Geometry: final body of the model. Coordinates: model frame, mm. A direction names the side the tool comes from. Round coordinates to 2 decimals unless told otherwise and drop trailing zeros. Loops run counter-clockwise (first coordinate to the right, second up) from the corner with the lowest first, then second, coordinate; pieces in that order, holes last. Notation, with made-up numbers: M -29.5,13 L -13.5,13 A18 ccw -13.5,30 Z; hole C -3.75,26 d2. An arc over 180 degrees is marked long. Answer as a JSON object with one key per item and string values.
```python
from build123d import *

# Parameters (mm, degrees)
F1_DEPTH = 1.5
F3_DEPTH = 1
F4_R     = 1.3
F5_DEPTH = 25


with BuildPart() as f1:
    # F0 (on Top) → F1 (new body)
    with BuildSketch(Plane.XY):
        with BuildLine():
            Line((-2, 0), (0, 0))
            Line((0, 0), (2, 0))
            ThreePointArc((2, 0), (2.8640349955, 2.0859650045), (4.95, 2.95))
            Line((4.95, 2.95), (-4.95, 2.95))
            ThreePointArc((-4.95, 2.95), (-2.8640349955, 2.0859650045), (-2, 0))
        make_face()
        with BuildLine():
            Line((2, 0), (0, 0))
            Line((0, 0), (-2, 0))
            ThreePointArc((-2, 0), (-2.8640349955, -2.0859650045), (-4.95, -2.95))
            Line((-4.95, -2.95), (4.95, -2.95))
            ThreePointArc((4.95, -2.95), (2.8640349955, -2.0859650045), (2, 0))
        make_face()
        with BuildLine():
            ThreePointArc((4.95, 2.95), (2.8640349955, 2.0859650045), (2, 0))
            Line((2, 0), (4.95, 0))
            Line((4.95, 0), (4.95, 2.95))
        make_face()
        with BuildLine():
            Line((4.95, 0), (2, 0))
            ThreePointArc((2, 0), (2.8640349955, -2.0859650045), (4.95, -2.95))
            ThreePointArc((4.95, -2.95), (7.0359650045, -2.0859650045), (7.9, 0))
            ThreePointArc((7.9, 0), (7.0359650045, 2.0859650045), (4.95, 2.95))
            Line((4.95, 2.95), (4.95, 0))
        make_face()
        with BuildLine():
            ThreePointArc((-4.95, -2.95), (-2.8640349955, -2.0859650045), (-2, 0))
            ThreePointArc((-2, 0), (-2.8640349955, 2.0859650045), (-4.95, 2.95))
            ThreePointArc((-4.95, 2.95), (-7.9, 0), (-4.95, -2.95))
        make_face()
    extrude(amount=F1_DEPTH)

    # F2 (on face) → F3 (cut)
    with BuildSketch(Plane(origin=(0, 0, 0), x_dir=(1, 0, 0), z_dir=(0, 0, -1))):
        Polygon((1.3, -2.2516660498), (2.6, 0), (1.3, 2.2516660498), (-1.3, 2.2516660498), (-2.6, 0), (-1.3, -2.2516660498), align=None)
    extrude(amount=-F3_DEPTH, mode=Mode.SUBTRACT)

    # F4 (on face) → F5 (cut)
    with BuildSketch(Plane(origin=(0, 0, 1), x_dir=(1, 0, 0), z_dir=(0, 0, -1))):
        Circle(F4_R)
    extrude(amount=-F5_DEPTH, mode=Mode.SUBTRACT)


solid = f1.part
```
1) Cut plane A-A on z = 0.35. Return the cut outline in (x, y).
Geometry results:
{"outline": "M -4.95,-2.95 L 4.95,-2.95 A2.95 ccw 4.95,2.95 L -4.95,2.95 A2.95 ccw Z; hole M -2.6,0 L -1.3,-2.25 L 1.3,-2.25 L 2.6,0 L 1.3,2.25 L -1.3,2.25 Z"}
2) Line query: probe 1 along X at (y, z) = (0, 1.45); probe 2 along Y at (x, z) = (0, 1.35); probe 3 along Y at (x, z) = (1, 0.95). Output: solid intervals per line, ascending.
Geometry results:
{"probe 1": "-7.9 to -1.3, 1.3 to 7.9", "probe 2": "-2.95 to -1.3, 1.3 to 2.95", "probe 3": "-2.95 to -2.25, 2.25 to 2.95"}
3) Cut plane C-C on y = 0.3. Return the cut outline in (x, z).
Geometry results:
{"outline": "M -7.88,0 L -2.43,0 L -2.43,1 L -1.26,1 L -1.26,1.5 L -7.88,1.5 Z; M 1.26,1 L 2.43,1 L 2.43,0 L 7.88,0 L 7.88,1.5 L 1.26,1.5 Z"}
4) Pull-direction query (Y, two-part tool) for faces 1 (the face through (0, 2.95, 1)), 2 (the face through (0, -2.95, 1)), 3 (the face through (1.96, -1.11, 0.49)), 4 (the face through (7.9, -0.1, 0.7)); classes: +Y half, -Y half, draft (parallel to the pull), parting line (faces both ways), or undercut.
Geometry results:
{"face 1": "+Y half", "face 2": "-Y half", "face 3": "undercut", "face 4": "parting line"}
5) Set-up query: faces 5 (the face through (1.94, 1.14, 0.49)), 6 (the face through (2, -2, 0)). Return all of +Z, -Z, +X, -X, +Y, -Y with unobstructed straight access to the full face (end or side cutting, diameter ignored); none if empty.
Geometry results:
{"face 5": "-Z", "face 6": "-Z, +X, -X, +Y, -Y"}
6) Cut plane D-D on x = -2. Return the cut outline in (y, z), and give its area (3 significant figures).
Geometry results:
{"outline": "M -2.95,0 L -1.04,0 L -1.04,1 L 1.04,1 L 1.04,0 L 2.95,0 L 2.95,1.5 L -2.95,1.5 Z", "area": "6.77 mm2"}
7) Cut plane B-B on x = 0. Return the cut outline in (y, z), and give its area (3 significant figures).
Geometry results:
{"outline": "M -2.95,0 L -2.25,0 L -2.25,1 L -1.3,1 L -1.3,1.5 L -2.95,1.5 Z; M 1.3,1 L 2.25,1 L 2.25,0 L 2.95,0 L 2.95,1.5 L 1.3,1.5 Z", "area": "3.05 mm2"}
8) First-contact query: pin 1 (2 mm diameter, centred on x = 0.5, y = -1, fed in from -Z). Flat tip, straight axial feed; report the tip coordinate or a pass-through.
Geometry results:
{"pin 1": "z = 1"}
